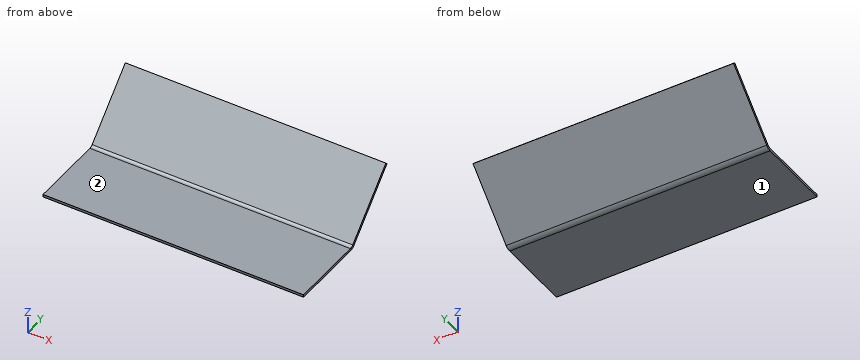
Autodesk Inventor part; units mm, degrees
ref_plane "YZ Plane" through (0, 0, 0) normal (1, 0, 0) x (0, 1, 0)
ref_plane "XZ Plane" through (0, 0, 0) normal (0, 1, 0) x (-1, 0, 0)
ref_plane "XY Plane" through (0, 0, 0) normal (0, 0, 1) x (1, 0, 0)
sketch "Sketch1" plane through (0, 0, 0) normal (0, 0, 1) x (1, 0, 0)
  line L0 (0, 0) -> (1000, 0)
  line L1 (1000, 0) -> (1000, 300)
  line L2 (1000, 300) -> (0, 300)
  line L3 (0, 300) -> (0, 0)
  dimension "d0" = 1000
  dimension "d1" = 300
extrude "Plate1" add sketch "Sketch1" along normal blind 10
sketch "Sketch2" plane through (0, 292.9289, 7.0711) normal (0, 0.7071068, -0.7071068) x (-1, 0, 0)
  line L0 (-1000, 0) -> (0, 0)
  line L1 (0, 0) -> (0, 300)
  line L2 (0, 300) -> (-1000, 300)
  line L3 (-1000, 300) -> (-1000, 0)
edge flange "Flange1" height 300 angle 45 thickness 10 bend radius 20 thickness toward (0, 0.7071068, -0.7071068) relief tear relief width 10 relief depth 5 edges at (500, 300, 10) wall of the first edge with corners at (1000, 292.9289, 7.0711) (0, 292.9289, 7.0711) (0, 505.061, 219.2031) (1000, 505.061, 219.2031)
bend "Bend1"
corner "Corner1"
equation "\"d2\" = Thickness"
equation "\"d3\" = BendReliefWidth"
equation "\"d4\" = BendReliefDepth"
equation "\"d5\" = MinimumRemnant"
equation "\"d6\" = TransitionRadius"
equation "\"d10\" = CornerReliefSize"
equation "\"d11\" = GapSize"
equation "\"d12\" = JacobiRadiusSize"
equation "\"BendReliefDepth\" = 0.5 * Thickness"
properties part number "10mm Polycarb Sheet" material "Polycarbonate, Clear"
Part model, mm, in its own coordinate system. Face numbers are marked on the shaded views. A direction names the side the tool comes from. Round coordinates to 2 decimals unless told otherwise and drop trailing zeros. Order: outer loops, then holes, each group sorted by start corner. A loop starts at its lowest first (then second) coordinate and runs counter-clockwise, first axis right, second up. Notation, with made-up numbers: M -22,36 L 4,36 A13 ccw 4,52 Z; hole C 39.5,-20.75 d9. An arc over 180 degrees is marked long. Answer in a Markdown table with one row per item. Add a question column.
Q1. 3-axis set-ups, long thin cutter, end or side, ignore diameter. For the marked faces 1 and 2: which of +Z, -Z, +X, -X, +Y, -Y reach the whole face in a straight line?
Q2. Cut at A-A on x = 420.5. Give the cut face in (y, z), and give its area (3 significant figures).
Q3. Cut at C-C on z = 60. Give the cut face in (x, y).
Q4. Pin check, flat tips, straight feed: pin 1 (2 mm diameter, centred on x = 671, z = 99.5, fed in from +Y); pin 2 (3 mm diameter, centred on x = 251.5, y = 279, fed in from +Z); pin 3 (12 mm diameter, centred on x = 665.5, z = 132, fed in from +Y). Stop position of each tip, or through.
Q5. Cut at B-B on y = 123.5. Give the cut face in (x, z), and give its area (3 significant figures).
Q6. Wall check: L1, parallel to Z at x = 744.5, y = 125.5; L2, parallel to Z at x = 474, y = 447; L3, parallel to Y at x = 677, z = 83.5. Give the ranges that are in metal, low to high. Write a range as from..to.
Established:
| question | item | result |
|---|---|---|
| 1 | face 1 | -Z, +X, -X, +Y, -Y |
| 1 | face 2 | +Z, +X, -X, -Y |
| 2 | outline | M 0,0 L 287.57,0 A30 ccw 308.79,8.79 L 512.13,212.13 L 505.06,219.2 L 301.72,15.86 A20 cw 287.57,10 L 0,10 Z |
| 2 | area | 5,950 mm2 |
| 3 | outline | M 0,345.86 L 1000,345.86 L 1000,360 L 0,360 Z |
| 4 | pin 1 | stops at y = 400.5 |
| 4 | pin 2 | stops at z = 10 |
| 4 | pin 3 | stops at y = 438 |
| 5 | outline | M 0,0 L 1000,0 L 1000,10 L 0,10 Z |
| 5 | area | 10,000 mm2 |
| 6 | L1 | z = 0..10 |
| 6 | L2 | z = 147..161.14 |
| 6 | L3 | y = 369.36..383.5 |
